```python
from build123d import *

# Parameters (mm, degrees)
SKETCH1_R           = 38.1
BOSS_EXTRUDE1_DEPTH = 10
SKETCH2_R           = 9.525
CUT_EXTRUDE1_DEPTH  = 6.35
SKETCH3_R           = 36.83
SKETCH3_R_2         = 11.1125
SKETCH3_R_3         = 11.115
CUT_EXTRUDE2_DEPTH  = 7.62


with BuildPart() as part:
    # Sketch1 → Boss-Extrude1 (new body)
    with BuildSketch(Plane(origin=(0, 0, 0), x_dir=(1, 0, 0), z_dir=(0, 1, 0))):
        Circle(SKETCH1_R)
    extrude(amount=BOSS_EXTRUDE1_DEPTH)

    # Sketch2 → Cut-Extrude1 (cut)
    with BuildSketch(Plane(origin=(0, 10, 0), x_dir=(1, 0, 0), z_dir=(0, 1, 0))):
        with Locations((25, 0)):
            Circle(SKETCH2_R)
        with Locations((-25, 0)):
            Circle(SKETCH2_R)
        with Locations((0, 15)):
            Circle(SKETCH2_R)
    extrude(amount=-CUT_EXTRUDE1_DEPTH, mode=Mode.SUBTRACT)

    # Sketch3 → Cut-Extrude2 (cut)
    with BuildSketch(Plane(origin=(0, 10, 0), x_dir=(1, 0, 0), z_dir=(0, 1, 0))):
        Circle(SKETCH3_R)
        with Locations((0, 15)):
            Circle(SKETCH3_R_2, mode=Mode.SUBTRACT)
        with Locations((25, 0)):
            Circle(SKETCH3_R_3, mode=Mode.SUBTRACT)
        with Locations((-25, 0)):
            Circle(SKETCH3_R_3, mode=Mode.SUBTRACT)
    extrude(amount=-CUT_EXTRUDE2_DEPTH, mode=Mode.SUBTRACT)


solid = part.part
```
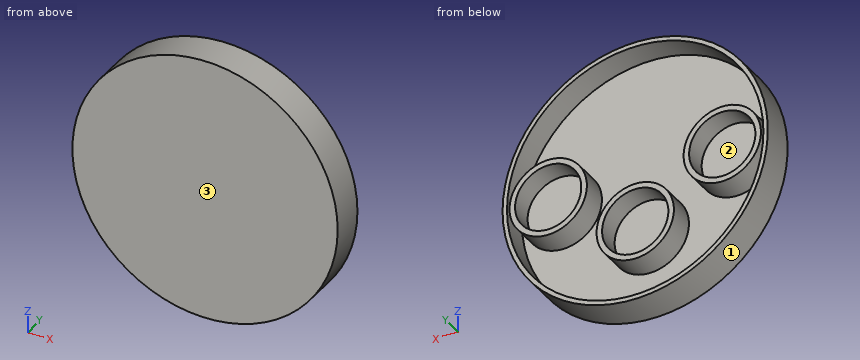
The model under review builds one solid part; all positions refer to its coordinate system, in mm. Face numbers are marked on the shaded views. Give positions to 0.01 mm unless a question says otherwise; leave off trailing zeros. Loops run counter-clockwise (first coordinate to the right, second up) from the corner with the lowest first, then second, coordinate; pieces in that order, holes last. Notation, with made-up numbers: (61.5, 40.25) - (100.5, 40.25) arc R10 cw to (100.5, 55.25) - close; hole circle Ø7 at (0, -23). An arc over 180 degrees is marked (long way). Answer as a JSON object with one key per item and string values.
Q1. Add section D-D on x = 19. State the section outline as (y, z) points, plus the area to 3 significant figures.
Worked out:
{"outline": "(0, -33.02) - (10, -33.02) - (10, -31.55) - (2.38, -31.55) - (2.38, -9.36) - (10, -9.36) - (10, -7.4) - (3.65, -7.4) - (3.65, 7.4) - (10, 7.4) - (10, 9.36) - (2.38, 9.36) - (2.38, 31.55) - (10, 31.55) - (10, 33.02) - (0, 33.02) - close", "area": "228 mm^2"}
Q2. Add section C-C on z = 0. State the section outline as (x, y) points (3 decimals), plus the area to 3 significant figures.
Worked out:
{"outline": "(-38.1, 0) - (38.1, 0) - (38.1, 10) - (36.83, 10) - (36.83, 2.38) - (36.115, 2.38) - (36.115, 10) - (34.525, 10) - (34.525, 3.65) - (15.475, 3.65) - (15.475, 10) - (13.885, 10) - (13.885, 2.38) - (-13.885, 2.38) - (-13.885, 10) - (-15.475, 10) - (-15.475, 3.65) - (-34.525, 3.65) - (-34.525, 10) - (-36.115, 10) - (-36.115, 2.38) - (-36.83, 2.38) - (-36.83, 10) - (-38.1, 10) - close", "area": "298 mm^2"}
Q3. Add section A-A on y = 5.5. Count the separate pieces of the cut face and the enclosed holes in it, plus the area to 3 significant figures.
Worked out:
{"separate pieces": "4", "enclosed holes": "4", "area": "608 mm^2"}
Q4. Insertion check: pin 1 (6 mm diameter, centred on x = 14, z = 24.5, fed in from +Y); pin 2 (2 mm diameter, centred on y = 5, z = 19, fed in from +X); pin 3 (3 mm diameter, centred on x = 8.5, y = 2.5, fed in from +Z). Each pin has a flat end and moves straight along its axis. Give the tip position at first contact, or say it passes through.
Worked out:
{"pin 1": "stops at y = 2.38", "pin 2": "stops at x = 33.58", "pin 3": "stops at z = 37.45"}
Q5. Mouldability with a two-part tool opening along Z and no side actions: class the marked faces 1, 2 and 3 as +Z half, -Z half, draft (parallel to the pull), parting line (faces both ways), or undercut.
Worked out:
{"face 1": "parting line", "face 2": "undercut", "face 3": "draft"}
Q6. To check wall thickness, follow line 1 along X through (y, z) = (5, 0) (3 decimals); line 2 along Z through (x, y) = (0, 6.25) (1 decimal); line 3 along Z through (x, y) = (-25, 6.25) (3 decimals). State the ranges of each line that lie inside material, in increasing order.
Worked out:
{"line 1": "x = -38.1 to -36.83, -36.115 to -34.525, -15.475 to -13.885, 13.885 to 15.475, 34.525 to 36.115, 36.83 to 38.1", "line 2": "z = -38.1 to -36.8, -26.1 to -24.5, -5.5 to -3.9, 36.8 to 38.1", "line 3": "z = -28.751 to -27.045, -11.115 to -9.525, 9.525 to 11.115, 27.045 to 28.751"}
